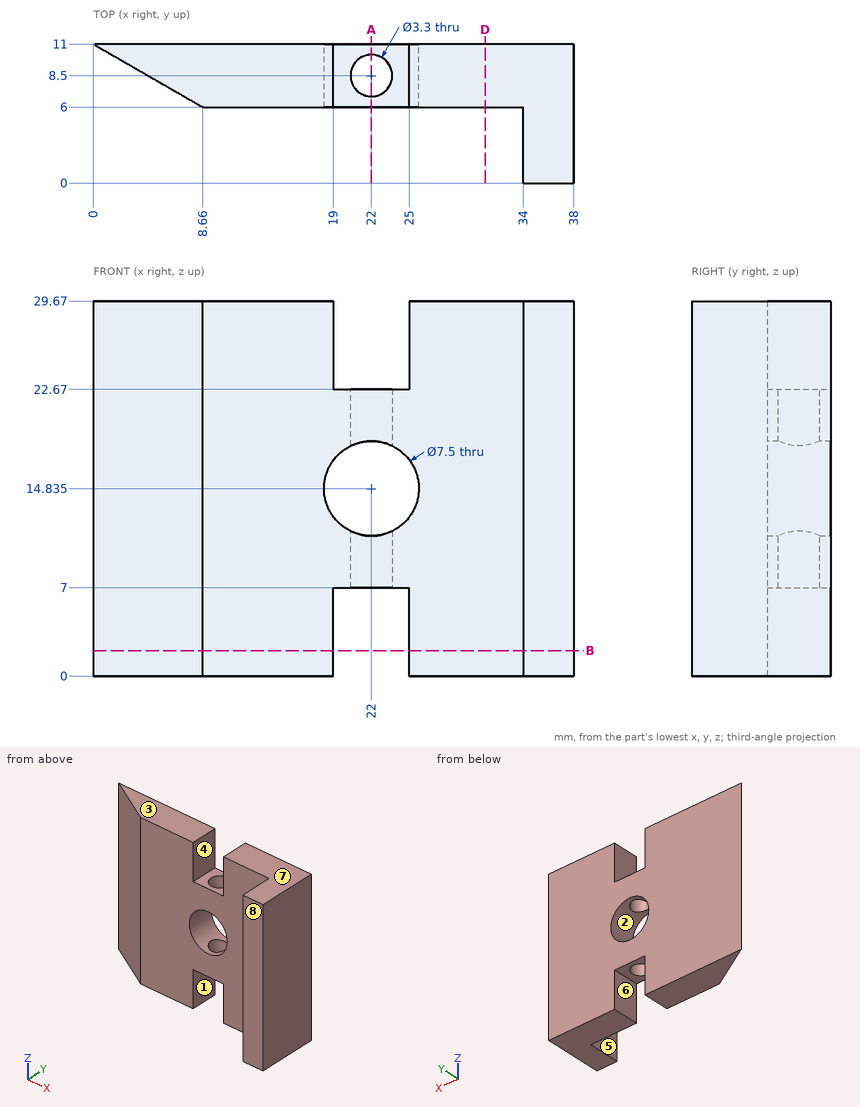
Verification items for this drawing (mm, ordinates from the low corner). A direction names the side the tool comes from. Coordinates: 2 decimals unless noted, no trailing zeros. Order: outer loops, then holes, each group sorted by start corner. A loop starts at its lowest first (then second) coordinate and runs counter-clockwise, first axis right, second up. Notation, with made-up numbers: (-12.5, 84) - (20.5, 84) arc R32 ccw to (20.5, 111) - close; hole circle Ø6 at (8.25, 62). An arc over 180 degrees is marked (long way). Answer in a Markdown table with one row per item. Add a question column.
1. Gauge pin test, flat ends, axial feed: pin 1 Ø2.5 at (y, z) = (8, 3.5) entering from -X; pin 2 Ø5.5 at (y, z) = (9, 25) entering from -X; pin 3 Ø1.8 at (y, z) = (3, 17.5) entering from -X; pin 4 Ø7.5 at (x, z) = (24.5, 16) entering from -Y. Record the tip position at first contact, or that the pin passes through.
2. Material ranges on L1, parallel to Y at x = 22, z = 9.75; L2, parallel to X at y = 0.5, z = 10; L3, parallel to Y at x = 28.5, z = 22.25, recorded low to high. Write a range as [from, to].
3. Access from +Z, -Z, +X, -X, +Y, -Y to the whole of each face (thin tool, end or side, straight path). Record for the marked faces 4, 5, 6, 7 and 8.
4. Section check B-B (z = 2). Enter the section's corners in (x, y), plus the area to 3 significant figures.
5. Draft check along Z on the marked faces 1, 2 and 3. Enter one of: +Z half, -Z half, draft (parallel to the pull), parting line (faces both ways), or undercut.
6. Section check D-D (x = 31). Enter the section's corners in (y, z).
7. Section check A-A (x = 22). Give the number of separate pieces and of enclosed holes in the cut face, plus the area to 3 significant figures.
Data:
| question | item | result |
|---|---|---|
| 1 | pin 1 | stops at x = 3.03 |
| 1 | pin 2 | stops at x = 0 |
| 1 | pin 3 | stops at x = 34 |
| 1 | pin 4 | stops at y = 6 |
| 2 | L1 | y = [6, 6.85], [10.15, 11] |
| 2 | L2 | x = [34, 38] |
| 2 | L3 | y = [6, 11] |
| 3 | face 4 | +Z, +Y, -Y |
| 3 | face 5 | +Z, -Z, -X, -Y |
| 3 | face 6 | -Z, +Y, -Y |
| 3 | face 7 | +Z, +X, -X, +Y, -Y |
| 3 | face 8 | +Z, -Z, +X, -X, -Y |
| 4 | outline | (0, 11) - (8.66, 6) - (19, 6) - (19, 11) - close; (25, 6) - (34, 6) - (34, 0) - (38, 0) - (38, 11) - (25, 11) - close |
| 4 | area | 162 mm² |
| 5 | face 1 | draft |
| 5 | face 2 | undercut |
| 5 | face 3 | +Z half |
| 6 | outline | (6, 0) - (11, 0) - (11, 29.67) - (6, 29.67) - close |
| 7 | separate pieces | 4 |
| 7 | enclosed holes | 0 |
| 7 | area | 13.9 mm² |
